Design review of the part built by this model. Coordinates are the model's own, in mm. A direction names the side the tool comes from. Coordinates: 2 decimals unless noted, no trailing zeros. Order: outer loops, then holes, each group sorted by start corner. A loop starts at its lowest first (then second) coordinate and runs counter-clockwise, first axis right, second up. Notation, with made-up numbers: M 19.5,47.5 L 63.5,47.5 A11 cw 63.5,58.5 Z; hole C 1,81 d1. An arc over 180 degrees is marked long. Use CSV: the item, a comma, the result in double quotes.
Autodesk Inventor part; units mm, degrees
ref_plane "Work Plane1" through (29, 0, 0) normal (0, -1, 0) x (1, 0, 0)
ref_plane "YZ Plane" through (0, 0, 0) normal (1, 0, 0) x (0, 1, 0)
ref_plane "XZ Plane" through (0, 0, 0) normal (0, 1, 0) x (-1, 0, 0)
sketch "Sketch1" plane through (0, 0, 0) normal (0, 0, 1) x (1, 0, 0)
  line L0 (-0.5, 0) -> (12, 0)
  line L1 (12, 0) -> (12, 1)
  line L2 (12, 1) -> (1.0454, 1)
  line L3 (1.0454, 1) -> (0.7999, 1)
  line L4 (0.7999, 1) -> (0, 1)
  line L5 (0, 1) -> (0, 1.9)
  line L6 (0, 1.9) -> (-2, 1.9)
  line L7 (-2, 1.9) -> (-2, 0.866)
  line L8 (-2, 0.866) -> (-1, 0.866)
  line L9 (-1, 0.866) -> (-0.5, 0)
  line L10 (-4.8, 0) -> (14.8, 0)
  line L11 (0, -0.38) -> (0, 2.28)
  line L12 (1.0454, 1) -> (0, 1) construction
  dimension "d1" = 10.9546
  dimension "d2" = 0.2455
  dimension "d3" = 2
  dimension "d4" = 1
  dimension "d5" = 60
  dimension "d6" = 2
  dimension "d7" = 2
  dimension "d8" = 1.7321
  dimension "d9" = 3.8
  dimension "d26" = 12
revolve "Body" add sketch "Sketch1" angle 360 about axis through (-0.5, 0, 0) along (1, 0, 0)
sketch "Sketch2" plane through (-2, 0, 0) normal (-1, 0, 0) x (0, 0, 1)
  circle A0 centre (0, 0) radius 0.866
  line L0 (0, -2.66) -> (0, 2.66)
  line L1 (-2.66, 0) -> (2.66, 0)
  line L2 (0.866, 0) -> (0.433, -0.75)
  line L3 (0.433, -0.75) -> (-0.433, -0.75)
  line L4 (-0.433, -0.75) -> (-0.866, 0)
  line L5 (-0.866, 0) -> (-0.433, 0.75)
  line L6 (-0.433, 0.75) -> (0.433, 0.75)
  line L7 (0.433, 0.75) -> (0.866, 0)
extrude "Slot" add sketch "Sketch2" against normal up to next contours L7 A0 | A0 L2 | L6 L0 A0 | A0 L0 L3 | L0 L6 A0 | A0 L3 L0 | L4 A0 | A0 L5
fillet "Fillet1" radius 0.2 1 edges at (-2, -1.9, 0)
thread "Thread"
chamfer "Chamfer1" distance 0.2454 distance2 0.2454 1 edges at (12, -1, 0) measured on face at (12, -0.5392, -0.3309)
ref_plane "Work Plane1" through (29, 0, 0) normal (0, -1, 0) x (1, 0, 0)
fillet "Fillet2" radius 0.1 1 edges at (0, -1, 0)
equation "\"d30\" = R"
equation "\"d17\" = RR"
equation "\"d13\" = GEL"
equation "\"d15\" = -0.5 * SPD + 0.5 * GD"
equation "\"d16\" = GUL"
equation "\"d1\" = GEL"
equation "\"d3\" = KOH"
equation "\"d4\" = INTI"
equation "\"d6\" = GD"
equation "\"d7\" = BDM"
equation "\"d8\" = 1.1547 * SW"
equation "\"d9\" = KOD"
equation "\"d26\" = NLG"
equation "\"GD\" = NND"
equation "\"NLG\" = 12"
equation "\"GEL\" = 10.95462"
equation "\"KOD\" = 3.8"
equation "\"KOH\" = 2"
equation "\"INTI\" = 1"
equation "\"GAL\" = 0.61345 * PTC"
equation "\"GUL\" = 0.61345 * PTC"
equation "\"BDM\" = NND"
equation "\"SW\" = 1.5"
equation "\"RR\" = 0.2"
equation "\"SPD\" = 1.50924"
equation "\"R\" = 0.1"
equation "\"TOA\" = 30deg"
equation "\"THREADDIA\" = 2"
equation "\"PTC\" = 0.4"
equation "\"NND\" = 2"
equation "\"E0\" = 1.155 * SW"
equation "\"GD1\" = THREADDIA - 1.2269 * PTC"
properties part number "ANSI B18.3.1M - M2x0.4 x 12" material "Steel, Mild"
(1) For faces 5 (the face through (-1.5, -0.75, 0)), 6 (the face through (-2, 1, 0)), list the 3-axis set-ups (+Z, -Z, +X, -X, +Y, -Y) from which the entire face can be reached by the end or side of a thin tool; tool diameter is ignored.
The answers:
face 5,"-X"
face 6,"+Z, -Z, -X, +Y, -Y"
(2) The part is to be moulded in two halves that separate along Y. For faces 1 (the face through (-0.53, 0.05, -0.02)), 2 (the face through (6, 0, 1)), 3 (the face through (-1.5, 0.75, 0)), 4 (the face through (0, 1, -1)), say which applies: pulls with the +Y half, pulls with the -Y half, needs draft (parallel to the pull), parting line crosses it, or undercut.
The answers:
face 1,"undercut"
face 2,"parting line crosses it"
face 3,"undercut"
face 4,"needs draft"
(3) Add section A-A on x = 9.25. State the section outline as (y, z) points, and give its area (3 significant figures).
The answers:
outline,"C 0,0 d2"
area,"3.14 mm2"
(4) Wall thickness on probe 1 along X at (y, z) = (-0.6, 1.2); probe 2 along Z at (x, y) = (5, 0.35); probe 3 along Z at (x, y) = (7.5, 0.25): over which ranges is each line inside the solid? List them lowest first.
The answers:
probe 1,"x = -2 to 0"
probe 2,"z = -0.94 to 0.94"
probe 3,"z = -0.97 to 0.97"
